Source: CAD feature listing. Evaluate the final solid. Frame: model axes, mm. A direction names the side the tool comes from. Round coordinates to 2 decimals unless told otherwise and drop trailing zeros. Order: outer loops, then holes, each group sorted by start corner. A loop starts at its lowest first (then second) coordinate and runs counter-clockwise, first axis right, second up. Notation, with made-up numbers: (29.5, 86) - (86.5, 86) arc R28 cw to (86.5, 116) - close; hole circle Ø3 at (71, 82). An arc over 180 degrees is marked (long way). Put each result on its own line as item: value. Start each with the question number.
1) Contact query for flat-ended pins moving along their axis: P1, Ø1.5, axis at y = 11, z = 1.5, coming from the +X side; P2, Ø12, axis at x = -12, y = 16, coming from the -Z side; P3, Ø1, axis at x = 10.5, y = 8, coming from the -Z side; P4, Ø12, axis at x = -15.5, z = -7.5, coming from the +Y side. Output: stop coordinate, or through.
2) Section B-B on z = -5.5. Output: boundary loops of the cut face in (x, y), then the cut area to 3 significant figures.
3) Section A-A on x = 0. Output: boundary loops of the cut face in (y, z), then the cut area to 3 significant figures.
4) Section C-C on y = -4.5. Output: boundary loops of the cut face in (x, z).
5) Access query for faces 1 (the face through (0, -4, 18.186)), 2 (the face through (17, 0, -1)). Directions: +Z, -Z, +X, -X, +Y, -Y. A direction counts if a zero-diameter tool reaches every point of the face in a straight line with its end or side. Return the directions, or none.
6) Line query: probe 1 along X at (y, z) = (-5, 0); probe 2 along Z at (x, y) = (0, 13); probe 3 along Y at (x, z) = (-13, 13). Output: solid intervals per line, ascending. Write a range as [from, to].
7) Section D-D on x = -15.5. Output: boundary loops of the cut face in (y, z), then the cut area to 3 significant figures.
Autodesk Inventor part; units mm, degrees
ref_plane "YZ Plane" through (0, 0, 0) normal (1, 0, 0) x (0, 1, 0)
ref_plane "XZ Plane" through (0, 0, 0) normal (0, 1, 0) x (-1, 0, 0)
ref_plane "XY Plane" through (0, 0, 0) normal (0, 0, 1) x (1, 0, 0)
sketch "Sketch1" plane through (0, 0, 0) normal (0, 1, 0) x (-1, 0, 0)
  circle A0 centre (0, 0) radius 16.5
  circle A1 centre (0, 0) radius 11.5
  dimension "d0" = 33
  dimension "d1" = 23
extrude "tappedEnd" add sketch "Sketch1" along normal blind 21
thread "Thread1"
sketch "Sketch2" plane through (0, 0, 0) normal (0, -1, 0) x (1, 0, 0)
  circle A0 centre (0, 0) radius 21 construction
  line L0 (-10.5, 18.1865) -> (10.5, 18.1865)
  line L1 (10.5, 18.1865) -> (21, 0)
  line L2 (21, 0) -> (10.5, -18.1865)
  line L3 (10.5, -18.1865) -> (-10.5, -18.1865)
  line L4 (-10.5, -18.1865) -> (-21, 0)
  line L5 (-21, 0) -> (-10.5, 18.1865)
  circle A1 centre (0, 0) radius 11.5
  dimension "d6" = 42
extrude "hexBit" add sketch "Sketch2" along normal blind 8
sketch "Sketch3" plane through (0, -8, 0) normal (0, -1, 0) x (1, 0, 0)
  circle A0 centre (0, 0) radius 11.5
  circle A1 centre (0, 0) radius 16.5
  dimension "d9" = 33
extrude "Extrusion3" [suppressed]
properties part number "PVCConnectorFemale3_4inch" material "PVC-Piping"
Answer sheet:
1. P1: x = 16.48
1. P2: z = -15.37
1. P3: z = -13.12
1. P4: y = 21
2. outline: (-17.82, -8) - (-10.1, -8) - (-10.1, 21) - (-15.56, 21) - (-15.56, 0) - (-17.82, 0) - close; (10.1, -8) - (17.82, -8) - (17.82, 0) - (15.56, 0) - (15.56, 21) - (10.1, 21) - close
2. area: 353 mm^2
3. outline: (-8, -18.19) - (0, -18.19) - (0, -16.5) - (21, -16.5) - (21, -11.5) - (-8, -11.5) - close; (-8, 11.5) - (21, 11.5) - (21, 16.5) - (0, 16.5) - (0, 18.19) - (-8, 18.19) - close
3. area: 317 mm^2
4. outline: (-21, 0) - (-10.5, -18.19) - (10.5, -18.19) - (21, 0) - (10.5, 18.19) - (-10.5, 18.19) - close; hole circle Ø23 at (0, 0)
5. face 1: +Z, +X, -X, +Y, -Y
5. face 2: +Y
6. probe 1: [-21, -11.5], [11.5, 21]
6. probe 2: [-16.5, -11.5], [11.5, 16.5]
6. probe 3: [-8, 0]
7. outline: (-8, -9.53) - (0, -9.53) - (0, -5.66) - (21, -5.66) - (21, 5.66) - (0, 5.66) - (0, 9.53) - (-8, 9.53) - close
7. area: 390 mm^2
